Autodesk Inventor part; units mm, degrees
ref_plane "YZ Plane" through (0, 0, 0) normal (1, 0, 0) x (0, 1, 0)
ref_plane "XZ Plane" through (0, 0, 0) normal (0, 1, 0) x (-1, 0, 0)
ref_plane "XY Plane" through (0, 0, 0) normal (0, 0, 1) x (1, 0, 0)
sketch "Szkic1" plane through (0, 0, 0) normal (0, 0, 1) x (1, 0, 0)
  line L0 (-6, -4) -> (6, -4)
  line L1 (6, 4) -> (-6, 4)
  line L2 (-6, 4) -> (-6, 2.5)
  line L3 (-6, 2.5) -> (-4.5, 2.5)
  line L4 (-4.5, 2.5) -> (-4.5, 1)
  line L5 (-4.5, 1) -> (-6, 1)
  line L6 (-6, 4) -> (-6, 2.5)
  line L7 (-6, 1) -> (-6, -4)
  line L8 (6, 4) -> (6, 2.5)
  line L9 (6, 2.5) -> (4.5, 2.5)
  line L10 (4.5, 2.5) -> (4.5, 1)
  line L11 (4.5, 1) -> (6, 1)
  line L12 (6, -4) -> (6, 1)
  line L13 (6, 2.5) -> (6, 4)
  point P0 (0, 0)
  dimension "d0" = 12
  dimension "d1" = 8
extrude "Wyciągnięcie proste1" add sketch "Szkic1" along normal blind 600
sketch "Szkic2" plane through (-6, 4, 600) normal (0, 1, 0) x (1, 0, 0)
  line L0 (12, 600) -> (0, 600)
  line L1 (0, 600) -> (0, 0)
  line L2 (12, 0) -> (0, 0)
  line L3 (12, 600) -> (12, 0)
  line L4 (6, 600) -> (6, 0)
  line L5 (0, 0) -> (12, 0)
  line L6 (6, 0) -> (6, 25)
  circle A0 centre (6, 25) radius 1.75
  dimension "d10" = 25
  dimension "d11" = 3.5
extrude "Wyciągnięcie proste2" cut sketch "Szkic2" against normal up to next contours A0 L4 | L4 A0
sketch "Szkic3" plane through (-6, 4, 600) normal (0, 1, 0) x (1, 0, 0)
  circle A0 centre (6, 25) radius 1.75
  circle A1 centre (6, 25) radius 3
  point P0 (6, 600)
  dimension "d14" = 6
extrude "Wyciągnięcie proste3" cut sketch "Szkic3" against normal blind 4.5
pattern_linear "Szyk prostokątny1" count 23 spacing 25 along (0, 0, -1) of "Wyciągnięcie proste2"
pattern_linear "Szyk prostokątny2" count 23 spacing 25 along (0, 0, -1) of "Wyciągnięcie proste3"
properties part number "Prowadnica liniowa typu MGN12H 600mm"
The model under review builds one solid part; all positions refer to its coordinate system, in mm. Give positions to 0.01 mm unless a question says otherwise; leave off trailing zeros. Write each loop counter-clockwise with the first axis right and the second up, starting at its lowest first coordinate (ties: lowest second). Pieces come first, ordered by that corner, then holes. Notation, with made-up numbers: (89, 73.25) - (100, 73.25) arc R23 cw to (100, 81.25) - close; hole circle Ø1 at (70.25, -27). An arc over 180 degrees is marked (long way). Answer in a Markdown table with one row per item. Add a question column.
1. Insertion check: P1, Ø5, axis at x = 0, z = 175, coming from the +Y side; P2, Ø3, axis at x = 0, z = 500, coming from the +Y side. Each pin has a flat end and moves straight along its axis. Give the tip position at first contact, or say it passes through.
2. Wall thickness on line 1 along X through (y, z) = (2.2, 275); line 2 along X through (y, z) = (-1.9, 525); line 3 along Y through (x, z) = (-5, 399): over which ranges is each line inside the solid? List them lowest first. Write a range as [from, to].
3. We need section A-A on z = 40.5. Write out the cut boundary in (x, y), then the cut area to 3 significant figures.
Ans:
| question | item | result |
|---|---|---|
| 1 | P1 | stops at y = -0.5 |
| 1 | P2 | passes through |
| 2 | line 1 | x = [-4.5, -3], [3, 4.5] |
| 2 | line 2 | x = [-6, -1.75], [1.75, 6] |
| 2 | line 3 | y = [-4, 1], [2.5, 4] |
| 3 | outline | (-6, -4) - (6, -4) - (6, 1) - (4.5, 1) - (4.5, 2.5) - (6, 2.5) - (6, 4) - (-6, 4) - (-6, 2.5) - (-4.5, 2.5) - (-4.5, 1) - (-6, 1) - close |
| 3 | area | 91.5 mm^2 |
